Geometry check sheet. Reference: the model listing, model coordinates, mm. A direction names the side the tool comes from. Give positions to 0.01 mm unless a question says otherwise; leave off trailing zeros. Write each loop counter-clockwise with the first axis right and the second up, starting at its lowest first coordinate (ties: lowest second). Pieces come first, ordered by that corner, then holes. Notation, with made-up numbers: (11, 57) -> (20, 57) arc R32 cw to (20, 90) -> close; hole circle Ø11 at (17, 56.25). An arc over 180 degrees is marked (long way). One line per item, written item: value.
from build123d import *

# Parameters (mm, degrees)
F0_W     = 41.8783635832
F0_H     = 39.4817627966
F1_DEPTH = 76.2
F3_DEPTH = 76.2
F5_DEPTH = 36.195
F7_DEPTH = 76.2


with BuildPart() as f1:
    # F0 (on Front) → F1 (new body)
    with BuildSketch(Plane.XZ):
        with Locations((-28.6883309018, 41.6107345372)):
            Rectangle(F0_W, F0_H)
    extrude(amount=F1_DEPTH)

    # F2 (on face) → F3 (cut)
    with BuildSketch(Plane.YZ.offset(-7.7491491102)):
        Polygon((0, 21.8698531389), (-39.980173111, 44.6278005838), (-39.980173111, 21.8698531389), align=None)
    extrude(amount=-F3_DEPTH, mode=Mode.SUBTRACT)

    # F4 (on face) → F5 (join)
    with BuildSketch(Plane(origin=(0, -39.980173111, 0), x_dir=(-1, 0, 0), z_dir=(0, 1, 0))):
        with BuildLine():
            Line((49.6275126934, 21.8698531389), (7.7491491102, 21.8698531389))
            ThreePointArc((7.7491491102, 21.8698531389), (28.6883309018, 0.9306713473), (49.6275126934, 21.8698531389))
        make_face()
    extrude(amount=-F5_DEPTH)

    # F6 (on face) → F7 (cut)
    with BuildSketch(Plane.YZ.offset(-7.7491491102)):
        Polygon((0, 44.6278005838), (-39.980173111, 44.6278005838), (0, 21.8698531389), align=None)
    extrude(amount=-F7_DEPTH, mode=Mode.SUBTRACT)


solid = f1.part
1) Sectioned sample at C-C on z = 43. Record the cut outline in (x, y), plus the area to 3 significant figures.
Verdict:
outline: (-49.63, -76.2) -> (-7.75, -76.2) -> (-7.75, -39.98) -> (-49.63, -39.98) -> close
area: 1,520 mm^2
2) Scan lines: probe 1 along Z at (x, y) = (-42, -34); probe 2 along Y at (x, z) = (-28, 14); probe 3 along Z at (x, y) = (-46.5, -57). Record each from-to range of solid material in increasing order.
Verdict:
probe 1: 44.63 to 61.35
probe 2: -76.18 to -39.98
probe 3: 10.86 to 61.35
3) Depth check by flat-ended pin: pin 1 Ø21 at (x, z) = (-23, 31) entering from +Y. Enter the tip coordinate at first touch or a pass-through.
Verdict:
pin 1: y = -39.98
4) Tool access check on faces 1 (the flat face through (-29, 0, 53)), 2 (the flat face through (-28, -39.98, 23)). Record the directions out of +Z, -Z, +X, -X, +Y, -Y that give a thin tool (end or side, any length) a straight path to the whole face; none if there is none.
Verdict:
face 1: +Z, -Z, +X, -X, +Y
face 2: -Z, +X, -X, +Y
5) Sectioned sample at B-B on y = -24. Record the cut outline in (x, z).
Verdict:
outline: (-49.63, 44.63) -> (-7.75, 44.63) -> (-7.75, 61.35) -> (-49.63, 61.35) -> close
